Work out the finished part from the listing and answer in its coordinate system (mm). A direction names the side the tool comes from. Give positions to 0.01 mm unless a question says otherwise; leave off trailing zeros. Loops run counter-clockwise (first coordinate to the right, second up) from the corner with the lowest first, then second, coordinate; pieces in that order, holes last. Notation, with made-up numbers: (8.25, 42.25) - (32.25, 42.25) arc R17 cw to (32.25, 73.25) - close; hole circle Ø9 at (2, -9). An arc over 180 degrees is marked (long way). One line per question, with ' | ' between items. Start each with the question number.
1. Which of the six approach directions +Z, -Z, +X, -X, +Y, -Y give full straight-line access (tool end or side, diameter ignored) to faces 1 (the face through (2.17, 151.48, -9.76)), 2 (the face through (10, -9.9, 3.2)), 3 (the face through (2, -20, -7)), 4 (the face through (0, 150, 8.2))?
2. Section B-B (y = -58.5) is taken. Determine the outline of the cut face in (x, z).
3. Each of these flat-tipped pins is pushed along its axis until it touches: pin 1 (6 mm diameter, centred on x = -3, y = -37.5, fed in from +Z); pin 2 (2 mm diameter, centred on y = 127.5, z = -4, fed in from -X); pin 3 (5 mm diameter, centred on y = 128, z = 6, fed in from -X). Where does it stop, or does it pass through?
4. Find the intervals of material crossed by line 1 (Y direction, x = 0.25, z = 9.5); line 2 (Y direction, x = 4.5, z = -9); line 3 (X direction, y = 112, z = -0.5), in increasing order.
5. Section D-D (y = 105.5) is taken. Determine the outline of the cut face in (x, z).
6. For a pull along Y with two mould halves and no side action, classify faces 5 (the face through (1.73, 73.95, -7.81)), 6 (the face through (0, 153, 0)), 7 (the face through (0, -80, 0)) as released by +Y, released by -Y, zero draft, split by the parting line, or undercut.
7. Section A-A (x = 0) is taken. Determine the outline of the cut face in (y, z).
8. Section C-C (z = -3.5) is taken. Determine the outline of the cut face in (x, y).
from build123d import *

# Parameters (mm, degrees)
F0_R     = 10.5
F1_DEPTH = 20
F2_R     = 7
F3_DEPTH = 60
F4_R     = 8
F5_R     = 8
F6_DEPTH = 150
F7_R     = 10
F8_DEPTH = 3


with BuildPart() as f1:
    # F0 (on Front) → F1 (new body)
    with BuildSketch(Plane.XZ):
        Circle(F0_R)
    extrude(amount=F1_DEPTH)

    # F2 (on face) → F3 (join)
    with BuildSketch(Plane.XZ.offset(20)):
        Circle(F2_R)
    extrude(amount=F3_DEPTH)

    # F4 (on face) + F5 (on face) → F6 (join)
    with BuildSketch(Plane(origin=(0, 0, 0), x_dir=(-1, 0, 0), z_dir=(0, 1, 0))):
        Circle(F4_R)
    with BuildSketch(Plane(origin=(0, 0, 0), x_dir=(-1, 0, 0), z_dir=(0, 1, 0))):
        Circle(F5_R)
    extrude(amount=F6_DEPTH)

    # F7 (on face) → F8 (join)
    with BuildSketch(Plane(origin=(0, 150, 0), x_dir=(-1, 0, 0), z_dir=(0, 1, 0))):
        Circle(F7_R)
    extrude(amount=F8_DEPTH)


solid = f1.part
Conclusion:
1) face 1: +Y | face 2: +Y, -Y | face 3: -Y | face 4: none
2) outline: circle Ø14 at (0, 0)
3) pin 1: z = 7 | pin 2: x = -7.42 | pin 3: x = -7.19
4) line 1: -20 to 0, 150 to 153 | line 2: -20 to 0 | line 3: -7.98 to 7.98
5) outline: circle Ø16 at (0, 0)
6) face 5: undercut | face 6: released by +Y | face 7: released by -Y
7) outline: (-80, -7) - (-20, -7) - (-20, -10.5) - (0, -10.5) - (0, -8) - (150, -8) - (150, -10) - (153, -10) - (153, 10) - (150, 10) - (150, 8) - (0, 8) - (0, 10.5) - (-20, 10.5) - (-20, 7) - (-80, 7) - close
8) outline: (-9.9, -20) - (-6.06, -20) - (-6.06, -80) - (6.06, -80) - (6.06, -20) - (9.9, -20) - (9.9, 0) - (7.19, 0) - (7.19, 150) - (9.37, 150) - (9.37, 153) - (-9.37, 153) - (-9.37, 150) - (-7.19, 150) - (-7.19, 0) - (-9.9, 0) - close
